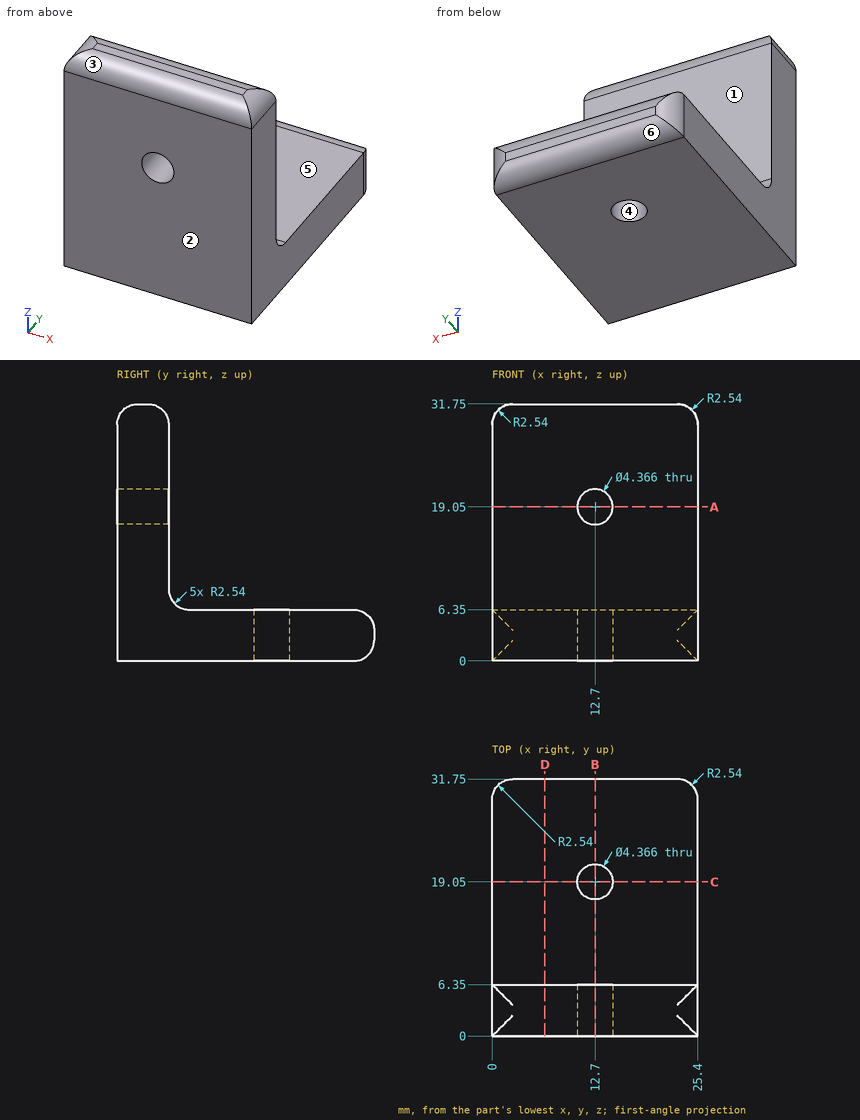
Input: dimensioned drawing with shaded views. Units: mm. Origin: part minimum x, y, z. A direction names the side the tool comes from. Coordinates: 2 decimals unless noted, no trailing zeros. Write each loop counter-clockwise with the first axis right and the second up, starting at its lowest first coordinate (ties: lowest second). Pieces come first, ordered by that corner, then holes. Notation, with made-up numbers: M 83,49.5 L 97,49.5 A15 ccw 97,55.5 Z; hole C 17,-38 d2. An arc over 180 degrees is marked long. Answer as a JSON object with one key per item and string values. Group by question number.
(1) Mould query, pull axis Y, two halves, no side actions, for the marked faces 3, 4, 5 and 6. Classes: pulls with the +Y half, pulls with the -Y half, needs draft (parallel to the pull), parting line crosses it, or undercut.
(2) Section A-A on z = 19.05. Output: boundary loops of the cut face in (x, y), plus the area to 3 significant figures.
(3) Contact query for flat-ended pins moving along their axis: P1, Ø7, axis at x = 12.7, y = 19.05, coming from the +Z side; P2, Ø10, axis at y = 13.5, z = 7, coming from the +X side; P3, Ø1.5, axis at x = 14, z = 22, coming from the +Y side; P4, Ø2.5, axis at x = 12.7, z = 19.05, coming from the -Y side. Output: stop coordinate, or through.
(4) Section D-D on x = 6.5. Output: boundary loops of the cut face in (y, z).
(5) Ray query, line 1 along X through (y, z) = (3.75, 19.05); line 2 along Y through (x, z) = (12.7, 3); line 3 along Y through (x, z) = (6.75, 21). Return the intervals inside material, ascending. Write a range as [from, to].
(6) Section B-B on x = 12.7. Output: boundary loops of the cut face in (y, z).
(7) Set-up query: the marked faces 1 and 2. Return all of +Z, -Z, +X, -X, +Y, -Y with unobstructed straight access to the full face (end or side cutting, diameter ignored); none if empty.
Result set:
{
 "1": {"face 3": "pulls with the -Y half", "face 4": "undercut", "face 5": "needs draft", "face 6": "pulls with the +Y half"},
 "2": {"outline": "M 0,0 L 10.52,0 L 10.52,6.35 L 0,6.35 Z; M 14.88,0 L 25.4,0 L 25.4,6.35 L 14.88,6.35 Z", "area": "134 mm2"},
 "3": {"P1": "stops at z = 6.35", "P2": "stops at x = 25.4", "P3": "stops at y = 6.35", "P4": "passes through"},
 "4": {"outline": "M 0,0 L 29.21,0 A2.54 ccw 31.75,2.54 L 31.75,3.81 A2.54 ccw 29.21,6.35 L 8.89,6.35 A2.54 cw 6.35,8.89 L 6.35,29.21 A2.54 ccw 3.81,31.75 L 2.54,31.75 A2.54 ccw 0,29.21 Z"},
 "5": {"line 1": "x = [0, 10.52], [14.88, 25.4]", "line 2": "y = [0, 16.87], [21.23, 31.75]", "line 3": "y = [0, 6.35]"},
 "6": {"outline": "M 0,0 L 16.87,0 L 16.87,6.35 L 8.89,6.35 A2.54 cw 6.35,8.89 L 6.35,16.87 L 0,16.87 Z; M 0,21.23 L 6.35,21.23 L 6.35,29.21 A2.54 ccw 3.81,31.75 L 2.54,31.75 A2.54 ccw 0,29.21 Z; M 21.23,0 L 29.21,0 A2.54 ccw 31.75,2.54 L 31.75,3.81 A2.54 ccw 29.21,6.35 L 21.23,6.35 Z"},
 "7": {"face 1": "+Z, +X, -X, +Y", "face 2": "+Z, -Z, +X, -X, -Y"}
}
